Check sheet for the modelled part. Datum: model origin and axes. Units: mm. Face numbers are marked on the shaded views. A direction names the side the tool comes from. Round coordinates to 2 decimals unless told otherwise and drop trailing zeros. Order: outer loops, then holes, each group sorted by start corner. A loop starts at its lowest first (then second) coordinate and runs counter-clockwise, first axis right, second up.
(1) Sectioned sample at D-D, the plane x = 15. Count the separate pieces of the cut face and the enclosed holes in it, and give its area (3 significant figures).
(2) Tool access check on the marked faces 1, 2, 3 and 4. Record the directions out of +Z, -Z, +X, -X, +Y, -Y that give a thin tool (end or side, any length) a straight path to the whole face; none if there is none.
(3) Sectioned sample at A-A, the plane z = 11.5. Enter the section's corners in (x, y), and give its area (3 significant figures).
(4) Mould release check, pull along X, two halves, no side actions. Record for the marked faces 5, 6, 7 and 8: released by +X, released by -X, zero draft, split by the parting line, or undercut.
(5) Sectioned sample at B-B, the plane z = -19. Enter the section's corners in (x, y).
(6) Sectioned sample at C-C, the plane z = 0. Enter the section's corners in (x, y).
(7) Depth check by flat-ended pin: pin 1 (3.5 mm diameter, centred on x = -3.5, z = -9, fed in from +Y); pin 2 (1.2 mm diameter, centred on x = -25.5, y = 12, fed in from +Z); pin 3 (1.1 mm diameter, centred on x = -13.5, y = 5, fed in from +Z). Enter the tip coordinate at first touch or a pass-through.
(8) Thickness scan on probe 1 along X at (y, z) = (13.75, -19); probe 2 along Y at (x, z) = (24, -12); probe 3 along X at (y, z) = (-1.5, -6.5). Record the ranges inside material, lowest first.
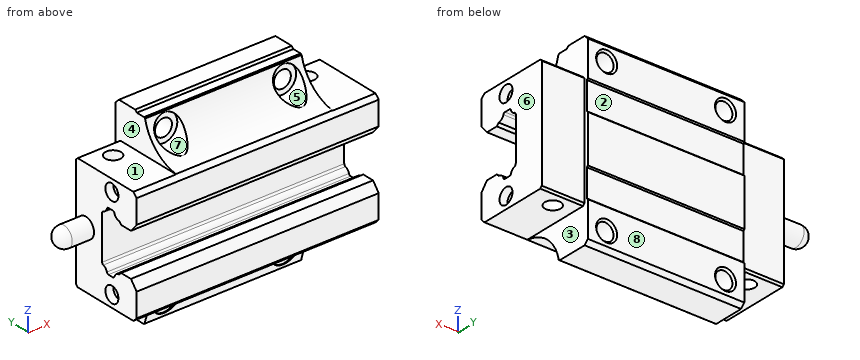
```python
from build123d import *

# Parameters (mm, degrees)
EXTRUDE_1_DEPTH          = 30.55
EXTRUDE_2_DEPTH          = 19.75
SKETCH_14_R              = 2.15
CUT_EXTRUDE_7_DEPTH      = 44.240172294
CUT_EXTRUDE_2_DEPTH      = 42.926155416
CUT_EXTRUDE_2_DEPTH_BACK = 42.926155416
SKETCH_13_R              = 2
CUT_EXTRUDE_6_DEPTH      = 2
SKETCH_16_R              = 1
CUT_EXTRUDE_11_DEPTH     = 5
SKETCH_12_R              = 2
CUT_EXTRUDE_5_DEPTH      = 5
SKETCH_15_R              = 3.5
CUT_EXTRUDE_10_DEPTH     = 10.7
CUT_EXTRUDE_8_DEPTH      = 58.918822542
CHAMFER_1_SIZE           = 0.47
CHAMFER_2_SIZE           = 0.26359415
CHAMFER_2_SIZE_2         = 0.24572937
CHAMFER_START            = -13
CHAMFER_3_OUTLINE_W      = 64
CHAMFER_3_OUTLINE_H      = 21.737972568
CHAMFER_3_DEPTH          = 1.262027432
CHAMFER_START_2          = 3.111269837
CHAMFER_3_2_DEPTH        = 24.465894629
CHAMFER_4_SIZE           = 0.5
FILLET_1_R               = 0.5


with BuildPart() as part:
    # 草图1 → 凸台-拉伸1 (new, symmetric)
    with BuildSketch(Plane(origin=(0, 0, 0), x_dir=(0, 0, -1), z_dir=(1, 0, 0))):
        with BuildLine():
            Line((-14.5, 15.5), (14.5, 15.5))
            Line((14.5, 15.5), (14.5, -3.1))
            Line((14.5, -3.1), (7.5, -3.1))
            Line((7.5, -3.1), (5.4, -1.35))
            Line((5.4, -1.35), (5.4, 1.65))
            Line((5.4, 1.65), (6, 2.25))
            ThreePointArc((6, 2.25), (6.439339828, 3.310660172), (7.5, 3.75))
            Line((7.5, 3.75), (7.5, 6))
            ThreePointArc((7.5, 6), (6.439339828, 6.439339828), (6, 7.5))
            Line((6, 7.5), (-6, 7.5))
            ThreePointArc((-6, 7.5), (-6.439339828, 6.439339828), (-7.5, 6))
            Line((-7.5, 6), (-7.5, 3.75))
            ThreePointArc((-7.5, 3.75), (-6.439339828, 3.310660172), (-6, 2.25))
            Line((-6, 2.25), (-5.4, 1.65))
            Line((-5.4, 1.65), (-5.4, -1.35))
            Line((-5.4, -1.35), (-7.5, -3.1))
            Line((-7.5, -3.1), (-14.5, -3.1))
            Line((-14.5, -3.1), (-14.5, 15.5))
        make_face()
    extrude(amount=EXTRUDE_1_DEPTH, both=True)

    # 草图2 → 凸台-拉伸2 (add, symmetric)
    with BuildSketch(Plane(origin=(0, 0, 0), x_dir=(0, 0, -1), z_dir=(1, 0, 0))):
        with BuildLine():
            Line((23.5, 7.6), (23.5, 15.5))
            Line((23.5, 15.5), (22.5, 16.5))
            Line((22.5, 16.5), (-22.5, 16.5))
            Line((-22.5, 16.5), (-23.5, 15.5))
            Line((-23.5, 15.5), (-23.5, 7.6))
            ThreePointArc((-23.5, 7.6), (-17.049167767, 3.890886925), (-14.5, -3.1))
            Line((-14.5, -3.1), (-14.5, 15.5))
            Line((-14.5, 15.5), (14.5, 15.5))
            Line((14.5, 15.5), (14.5, -3.1))
            ThreePointArc((14.5, -3.1), (17.049167767, 3.890886925), (23.5, 7.6))
        make_face()
    extrude(amount=EXTRUDE_2_DEPTH, both=True)

    # 草图14 → 切除-拉伸7 (cut, through all)
    with BuildSketch(Plane(origin=(0, 16.5, 0), x_dir=(1, 0, 0), z_dir=(0, 1, 0))):
        with Locations(Location((15, 19, 0), (0, 0, 270))):
            Circle(SKETCH_14_R)
        with Locations(Location((15, -19, 0), (0, 0, 270))):
            Circle(SKETCH_14_R)
        with Locations(Location((-15, -19, 0), (0, 0, 270))):
            Circle(SKETCH_14_R)
        with Locations(Location((-15, 19, 0), (0, 0, 270))):
            Circle(SKETCH_14_R)
    extrude(amount=-CUT_EXTRUDE_7_DEPTH, mode=Mode.SUBTRACT)

    # 草图5 → 切除-拉伸2 (cut, two sides: drawn at the far end of the back side and taken through both)
    with BuildSketch(Plane(origin=(0, 0, 0), x_dir=(0, 0, -1), z_dir=(1, 0, 0)).offset(-CUT_EXTRUDE_2_DEPTH_BACK)):
        Polygon((-23, 10), (-23, 7.1), (-23.5, 7.6), (-23.5, 10.5), align=None)
    extrude(amount=CUT_EXTRUDE_2_DEPTH + CUT_EXTRUDE_2_DEPTH_BACK, mode=Mode.SUBTRACT)

    # 草图18 → 旋转1 (revolve)
    with BuildSketch(Plane.XY):
        with BuildLine():
            Line((-30.55, 12.5), (-38.55, 12.5))
            ThreePointArc((-38.55, 12.5), (-37.817766953, 14.267766953), (-36.05, 15))
            Line((-36.05, 15), (-30.55, 15))
            Line((-30.55, 15), (-30.55, 12.5))
        make_face()
    revolve(axis=Axis((-30.55, 12.5, 0), (-1, 0, 0)))

    # 草图13 → 切除-拉伸6 (cut)
    with BuildSketch(Plane.ZY.offset(30.55)):
        with Locations((-11.5, 4.5)):
            Circle(SKETCH_13_R)
        with Locations(Location((11.5, 4.5, 0), (0, 0, 180))):
            Circle(SKETCH_13_R)
    cut_extrude_6 = extrude(amount=-CUT_EXTRUDE_6_DEPTH, mode=Mode.SUBTRACT)

    # 草图16 → 切除-拉伸11 (cut)
    with BuildSketch(Plane.ZY.offset(28.55)):
        with Locations((-11.5, 4.5)):
            Circle(SKETCH_16_R)
        with Locations((11.5, 4.5)):
            Circle(SKETCH_16_R)
    cut_extrude_11 = extrude(amount=-CUT_EXTRUDE_11_DEPTH, mode=Mode.SUBTRACT)

    # 镜向3: 切除-拉伸6, 切除-拉伸11 across plane
    add(cut_extrude_6.mirror(Plane(origin=(0, 0, 0), x_dir=(0, 0, 1), z_dir=(1, 0, 0))), mode=Mode.SUBTRACT)
    add(cut_extrude_11.mirror(Plane(origin=(0, 0, 0), x_dir=(0, 0, 1), z_dir=(1, 0, 0))), mode=Mode.SUBTRACT)

    # 草图12 → 切除-拉伸5 (cut)
    with BuildSketch(Plane.XY.offset(14.5)):
        with Locations((-24.5, 11.5)):
            Circle(SKETCH_12_R)
        with Locations(Location((24.5, 11.5, 0), (0, 0, 180))):
            Circle(SKETCH_12_R)
    cut_extrude_5 = extrude(amount=-CUT_EXTRUDE_5_DEPTH, mode=Mode.SUBTRACT)

    # 草图15 → 切除-拉伸10 (cut)
    with BuildSketch(Plane.XZ.offset(3.1)):
        with Locations(Location((15, 19, 0), (0, 0, 270))):
            Circle(SKETCH_15_R)
        with Locations(Location((15, -19, 0), (0, 0, 270))):
            Circle(SKETCH_15_R)
        with Locations(Location((-15, 19, 0), (0, 0, 270))):
            Circle(SKETCH_15_R)
        with Locations(Location((-15, -19, 0), (0, 0, 270))):
            Circle(SKETCH_15_R)
    extrude(amount=-CUT_EXTRUDE_10_DEPTH, mode=Mode.SUBTRACT)

    # 镜向4: 切除-拉伸5 across plane
    add(cut_extrude_5.mirror(Plane.XY), mode=Mode.SUBTRACT)

    # 草图3 → 切除-拉伸8 (cut, through all)
    with BuildSketch(Plane.ZY.offset(19.75)):
        Polygon((-6, 16.5), (-6.3, 16.2), (-13.3, 16.2), (-13.6, 16.5), align=None)
        Polygon((13.6, 16.5), (13.3, 16.2), (6.3, 16.2), (6, 16.5), align=None)
    extrude(amount=-CUT_EXTRUDE_8_DEPTH, mode=Mode.SUBTRACT)

    # 倒角1
    chamfer_1_edges = [part.edges().sort_by_distance(p)[0] for p in [
        (25.15, -3.1, 14.5),
        (25.15, 15.5, 14.5),
        (25.15, 15.5, -14.5),
        (25.15, -3.1, -14.5),
        (-25.15, -3.1, 14.5),
        (-25.15, 15.5, 14.5),
        (-25.15, 15.5, -14.5),
        (-25.15, -3.1, -14.5),
    ]]
    chamfer(chamfer_1_edges, length=CHAMFER_1_SIZE)

    # 倒角2
    # the kernel refuses this chamfer: 0.26359415, 0.24572937, 0.2 mm, written as the material it takes off along each edge
    with BuildSketch(Plane(origin=(-20.431376675, 7.500917151, 23), x_dir=(0, -0.22641410518634636, -0.97403113552528), z_dir=(1, 0, 0))) as chamfer_2_piece_1:
        with BuildLine():
            Line((0.201885125, 0), (-CHAMFER_2_SIZE * 0.226414105253, CHAMFER_2_SIZE * 0.974031135813))
            Line((-CHAMFER_2_SIZE * 0.226414105253, CHAMFER_2_SIZE * 0.974031135813), (0, 0))
            ThreePointArc((0, 0), (0.104706276, 0.000468459), (0.201885125, 0))
        make_face()
    extrude(amount=40.862753349, mode=Mode.SUBTRACT)
    with BuildSketch(Plane(origin=(-20.384576532, 7.6, -23.5), x_dir=(0, -0.18046272794534762, 0.9835818236539975), z_dir=(1, 0, 0))) as chamfer_2_piece_2:
        with BuildLine():
            Line((0.201885125, 0), (-CHAMFER_2_SIZE_2 * 0.180462727665, -CHAMFER_2_SIZE_2 * 0.983581822127))
            Line((-CHAMFER_2_SIZE_2 * 0.180462727665, -CHAMFER_2_SIZE_2 * 0.983581822127), (0, 0))
            ThreePointArc((0, 0), (0.104451114, -0.000468545), (0.201885125, 0))
        make_face()
    extrude(amount=40.769153064, mode=Mode.SUBTRACT)

    # 倒角3: read off the stored shape, not the designer's step
    # 倒角3 outline → 倒角3 (cut)
    with BuildSketch(Plane(origin=(0, 0, 0), x_dir=(1, 0, 0), z_dir=(0, 0.707106781186547, 0.707106781186548)).offset(CHAMFER_START)):
        with Locations((0, -0.868986284)):
            Rectangle(CHAMFER_3_OUTLINE_W, CHAMFER_3_OUTLINE_H)
    extrude(amount=CHAMFER_3_DEPTH, mode=Mode.SUBTRACT)

    # Chamfer 3 2 outline → Chamfer 3 2 (cut)
    with BuildSketch(Plane(origin=(0, 0, 0), x_dir=(1, 0, 0), z_dir=(0, 0.707106781186547, 0.707106781186548)).offset(CHAMFER_START_2)):
        Polygon((32, -11.737972568), (-32, -11.737972568), (-32, -12.112739162), (-19.75, -12.112739162), (-19.75, -14), (19.75, -14), (19.75, -12.112739162), (32, -12.112739162), align=None)
    extrude(amount=CHAMFER_3_2_DEPTH, mode=Mode.SUBTRACT)

    # 倒角4
    chamfer_4_edges = [part.edges().sort_by_distance(p)[0] for p in [
        (15, 16.5, -21.15),
        (15, 16.5, 16.85),
        (-15, 16.5, 16.85),
        (-15, 16.5, -21.15),
    ]]
    chamfer(chamfer_4_edges, length=CHAMFER_4_SIZE)

    # 圆角1
    fillet_1_edges = [part.edges().sort_by_distance(p)[0] for p in [
        (0, 3.75, -7.5),
        (0, 6, -7.5),
        (0, 7.5, -6),
        (0, 7.5, 6),
        (0, 6, 7.5),
        (0, 3.75, 7.5),
    ]]
    fillet(fillet_1_edges, radius=FILLET_1_R)


solid = part.part
```
Derived:
1. separate pieces: 3
1. enclosed holes: 0
1. area: 526 mm2
2. face 1: +Z, -X, +Y, -Y
2. face 2: +X, -X, +Y
2. face 3: +X, +Y
2. face 4: -X, +Y
3. outline: (-30.55, -3.1) - (30.55, -3.1) - (30.55, 2.5) - (28.55, 2.5) - (28.55, 3.5) - (23.55, 3.5) - (23.55, 5.5) - (28.55, 5.5) - (28.55, 6.5) - (30.55, 6.5) - (30.55, 15.5) - (19.75, 15.5) - (19.75, 16.2) - (-19.75, 16.2) - (-19.75, 15.5) - (-30.55, 15.5) - (-30.55, 6.5) - (-28.55, 6.5) - (-28.55, 5.5) - (-23.55, 5.5) - (-23.55, 3.5) - (-28.55, 3.5) - (-28.55, 2.5) - (-30.55, 2.5) - close; hole circle Ø4 at (-24.5, 11.5); hole circle Ø4 at (24.5, 11.5)
3. area: 1,100 mm2
4. face 5: undercut
4. face 6: released by +X
4. face 7: undercut
4. face 8: zero draft
5. outline: (-19.75, 5.7) - (-18.5, 5.7) - (-18.5, 7.6) - (-17.15, 7.6) - (-17.15, 16) - (-17.65, 16.5) - (-19.75, 16.5) - close; (-12.85, 7.6) - (-11.5, 7.6) - (-11.5, 5.7) - (11.5, 5.7) - (11.5, 7.6) - (12.85, 7.6) - (12.85, 16) - (12.35, 16.5) - (-12.35, 16.5) - (-12.85, 16) - close; (17.15, 7.6) - (18.5, 7.6) - (18.5, 5.7) - (19.75, 5.7) - (19.75, 16.5) - (17.65, 16.5) - (17.15, 16) - close
6. outline: (-36.05, 10) - (-30.55, 10) - (-30.55, 7.5) - (30.55, 7.5) - (30.55, 15.5) - (19.75, 15.5) - (19.75, 16.5) - (-19.75, 16.5) - (-19.75, 15.5) - (-30.55, 15.5) - (-30.55, 15) - (-36.05, 15) arc R2.5 ccw to start
7. pin 1: stops at y = 16.2
7. pin 2: stops at z = 9.5
7. pin 3: stops at z = 16.16
8. probe 1: x = -19.75 to -17.15, -12.85 to 12.85, 17.15 to 19.75
8. probe 2: y = -3.1 to 3.63, 5.37 to 9.56, 13.44 to 15.5
8. probe 3: x = -30.55 to 30.55
